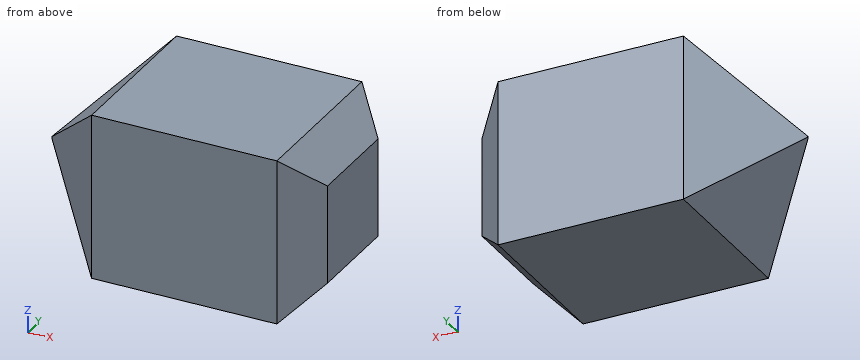
from build123d import *

# Parameters (mm, degrees)
SKETCH1_W           = 6.2865
SKETCH1_H           = 6.2865
BOSS_EXTRUDE1_DEPTH = 11.43
CHAMFER1_SIZE       = 1.27
CHAMFER2_SIZE       = 3.1115


with BuildPart() as part:
    # Sketch1 → Boss-Extrude1 (new body)
    with BuildSketch(Plane(origin=(0, 0, 0), x_dir=(0, 0, -1), z_dir=(1, 0, 0))):
        with Locations((3.14325, 3.14325)):
            Rectangle(SKETCH1_W, SKETCH1_H)
    extrude(amount=BOSS_EXTRUDE1_DEPTH)

    # Chamfer1
    chamfer1_edges = [part.edges().sort_by_distance(p)[0] for p in [
        (11.43, 3.14325, -6.2865),
        (11.43, 0, -3.14325),
        (11.43, 3.14325, 0),
        (11.43, 6.2865, -3.14325),
    ]]
    chamfer(chamfer1_edges, length=CHAMFER1_SIZE)

    # Chamfer2
    chamfer2_edges = [part.edges().sort_by_distance(p)[0] for p in [
        (0, 0, -3.14325),
        (0, 3.14325, -6.2865),
        (0, 6.2865, -3.14325),
        (0, 3.14325, 0),
    ]]
    chamfer(chamfer2_edges, length=CHAMFER2_SIZE)


solid = part.part
Source: CAD feature listing. Evaluate the final solid. Frame: model axes, mm. Coordinates: 2 decimals unless noted, no trailing zeros. Loops run counter-clockwise (first coordinate to the right, second up) from the corner with the lowest first, then second, coordinate; pieces in that order, holes last. Notation, with made-up numbers: (73, -26.5) -> (114, -26.5) arc R36 ccw to (114, 11.5) -> close; hole circle Ø4 at (81.5, -19). An arc over 180 degrees is marked (long way). Answer in a Markdown table with one row per item. Add a question column.
Q1. Contact query for a flat-ended pin moving along its axis: pin 1 Ø1 at (y, z) = (4, -5) entering from -X (3 decimals). Output: stop coordinate, or through.
Q2. Section B-B on y = 1. Return the cut outline in (x, z), and give its area (3 significant figures).
Q3. Section A-A on z = -2.25. Return the cut outline in (x, y), and give its area (3 significant figures).
Q4. Ray query, line 1 along Y through (x, z) = (2.25, -1.5) (1 decimal); line 2 along Y through (x, z) = (11, -4.5); line 3 along Z through (x, y) = (0.5, 3) (1 decimal). Return the intervals inside material, ascending.
Q5. Section D-D on x = 10.5. Return the cut outline in (y, z).
Q6. Section C-C on x = 1.25. Return the cut outline in (y, z) (1 decimal), and give its area (3 significant figures).
Computed values:
| question | item | result |
|---|---|---|
| 1 | pin 1 | stops at x = 1.325 |
| 2 | outline | (2.11, -5.29) -> (3.11, -6.29) -> (10.16, -6.29) -> (11.16, -5.29) -> (11.16, -1) -> (10.16, 0) -> (3.11, 0) -> (2.11, -1) -> close |
| 2 | area | 54.9 mm^2 |
| 3 | outline | (0.86, 2.25) -> (3.11, 0) -> (10.16, 0) -> (11.43, 1.27) -> (11.43, 5.02) -> (10.16, 6.29) -> (3.11, 6.29) -> (0.86, 4.04) -> close |
| 3 | area | 59.8 mm^2 |
| 4 | line 1 | y = 0.9 to 5.4 |
| 4 | line 2 | y = 0.84 to 5.45 |
| 4 | line 3 | z = -3.7 to -2.6 |
| 5 | outline | (0.34, -5.95) -> (5.95, -5.95) -> (5.95, -0.34) -> (0.34, -0.34) -> close |
| 6 | outline | (1.9, -4.4) -> (4.4, -4.4) -> (4.4, -1.9) -> (1.9, -1.9) -> close |
| 6 | area | 6.57 mm^2 |
